Can you work these out from the model? Positions are in its coordinate system, mm. A direction names the side the tool comes from. Give positions to 0.01 mm unless a question says otherwise; leave off trailing zeros. Order: outer loops, then holes, each group sorted by start corner. A loop starts at its lowest first (then second) coordinate and runs counter-clockwise, first axis right, second up.
Item 1: If I drill on line 1 along Y through (x, z) = (-29, 3.2); line 2 along Y through (x, z) = (-14.5, 11); line 3 along Y through (x, z) = (-19.5, 6.5), over which ranges is the centre line in solid material (lowest first)?
Item 2: I'm going to push flat-ended pins straight in: pin 1 Ø5 at (x, y) = (29.27, -29.27) entering from +Z; pin 2 Ø12 at (x, y) = (-8, -7.5) entering from +Z; pin 3 Ø5 at (x, z) = (-6, 14.5) entering from -Y. Where does each tip first touch, or does it pass through?
Item 3: I want a section at B-B, the plane y = 29. Write out the boundary of the cut face in (x, z).
Item 4: Which directions (+Z, -Z, +X, -X, +Y, -Y) give clear straight access to the entire face, cutting with the end or side of a thin tool? Please do faces 1 (the flat face through (-29, 29, 2.5)), 2 (the flat face through (0, -25, 13)), 3 (the flat face through (25, 0, 13)).
Item 5: I want a section at C-C, the plane z = 9. Write out the boundary of the cut face in (x, y), then the cut area to 3 significant figures.
Item 6: If we mould it in two halves opening along X, with no side actions, what happens to faces 4 (the cylindrical face through (-34, 33, 3)), 5 (the flat face through (20, 0, 15)), 6 (the flat face through (0, -35, 3)), 7 (the flat face through (35, 0, 3))? For each: +X half, -X half, draft (parallel to the pull), parting line (faces both ways), or undercut.
Item 7: I want a section at A-A, the plane x = -17.5. Write out the boundary of the cut face in (y, z), then the cut area to 3 significant figures.
```python
from build123d import *

# Parameters (mm, degrees)
F0_W     = 70
F0_H     = 70
F1_DEPTH = 5.2
F2_W     = 50
F2_H     = 50
F3_DEPTH = 15
F4_R     = 5
F5_R     = 2
F6_DEPTH = 2.7
F8_W     = 40
F8_H     = 40
F9_DEPTH = 10


# Not quite as in the source:
# - a feature names something its author has since deleted; it is built from what else it names


with BuildPart() as f1:
    # F0 (on Top) → F1 (new body)
    with BuildSketch(Plane.XY):
        Rectangle(F0_W, F0_H)
    extrude(amount=F1_DEPTH)

    # F2 (on face) → F3 (join)
    with BuildSketch(Plane.XY.offset(5.2)):
        Rectangle(F2_W, F2_H)
    extrude(amount=F3_DEPTH)

    # F4
    f4_edges = [f1.edges().sort_by_distance(p)[0] for p in [
        (-35, 35, 2.6),
        (35, 35, 2.6),
        (35, -35, 2.6),
        (-35, -35, 2.6),
    ]]
    fillet(f4_edges, radius=F4_R)

    # F5 (on face) → F6 (cut)
    with BuildSketch(Plane.XY.offset(5.2)):
        with Locations((-29, 29)):
            Circle(F5_R)
        with Locations((29.267766953, -29.267766953)):
            Circle(F5_R)
        with Locations((-29.267766953, -29.267766953)):
            Circle(F5_R)
    extrude(amount=-F6_DEPTH, mode=Mode.SUBTRACT)

    # F8 (on face) → F9 (cut)
    with BuildSketch(Plane.XY.offset(20.2)):
        Rectangle(F8_W, F8_H)
    extrude(amount=-F9_DEPTH, mode=Mode.SUBTRACT)


solid = f1.part
```
Results list:
1. line 1: y = -35 to -31.25, -27.29 to 27, 31 to 35
1. line 2: y = -25 to -20, 20 to 25
1. line 3: y = -25 to 25
2. pin 1: stops at z = 5.2
2. pin 2: stops at z = 10.2
2. pin 3: stops at y = -25
3. outline: (-35, 0) - (35, 0) - (35, 5.2) - (-27, 5.2) - (-27, 2.5) - (-31, 2.5) - (-31, 5.2) - (-35, 5.2) - close
4. face 1: +Z
4. face 2: +Z, +X, -X, -Y
4. face 3: +Z, +X, +Y, -Y
5. outline: (-25, -25) - (25, -25) - (25, 25) - (-25, 25) - close
5. area: 2,500 mm2
6. face 4: -X half
6. face 5: undercut
6. face 6: draft
6. face 7: +X half
7. outline: (-35, 0) - (35, 0) - (35, 5.2) - (25, 5.2) - (25, 20.2) - (20, 20.2) - (20, 10.2) - (-20, 10.2) - (-20, 20.2) - (-25, 20.2) - (-25, 5.2) - (-35, 5.2) - close
7. area: 714 mm2
